from build123d import *

# Parameters (mm, degrees)
BOSS_EXTRUDE1_DEPTH = 0.3
SKETCH2_R           = 0.085
CUT_EXTRUDE1_DEPTH  = 0.3


with BuildPart() as part:
    # Sketch1 → Boss-Extrude1 (new body)
    with BuildSketch(Plane(origin=(0, 0, 0), x_dir=(1, 0, 0), z_dir=(0, 1, 0))):
        with BuildLine():
            Line((0.284268307, -3), (-0.284268307, -3))
            Line((-0.284268307, -3), (-0.123615756, -0.587127878))
            ThreePointArc((-0.123615756, -0.587127878), (-0.6, 0), (-0.123615756, 0.587127878))
            Line((-0.123615756, 0.587127878), (-0.123615756, 14))
            Line((-0.123615756, 14), (0.123615756, 14))
            Line((0.123615756, 14), (0.123615756, 0.587127878))
            ThreePointArc((0.123615756, 0.587127878), (0.6, 0), (0.123615756, -0.587127878))
            Line((0.123615756, -0.587127878), (0.284268307, -3))
        make_face()
    extrude(amount=BOSS_EXTRUDE1_DEPTH)

    # Sketch2 → Cut-Extrude1 (cut)
    with BuildSketch(Plane(origin=(0, 0.3, 0), x_dir=(1, 0, 0), z_dir=(0, 1, 0))):
        Circle(SKETCH2_R)
    extrude(amount=-CUT_EXTRUDE1_DEPTH, mode=Mode.SUBTRACT)


solid = part.part
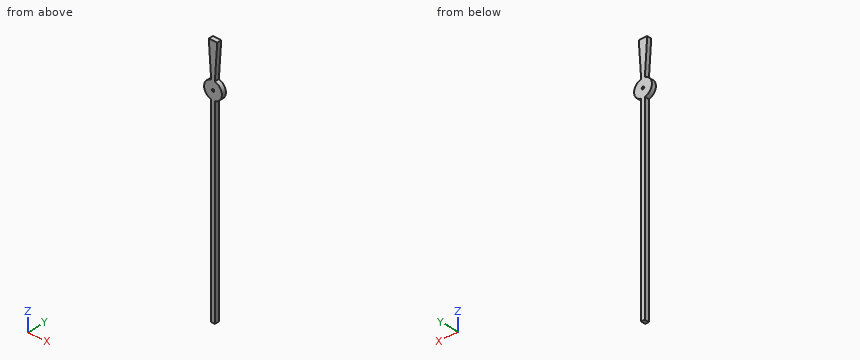
Check sheet for the modelled part. Datum: model origin and axes. Units: mm. Give positions to 0.01 mm unless a question says otherwise; leave off trailing zeros. Order: outer loops, then holes, each group sorted by start corner. A loop starts at its lowest first (then second) coordinate and runs counter-clockwise, first axis right, second up. Notation, with made-up numbers: M 44,79 L 100,79 A16 ccw 100,91 Z; hole C -28.5,-35 d6. An arc over 180 degrees is marked long. Answer as CSV lines item,"result". Start each with the question number.
Item 1: Cross-section at B-B on z = -9. Enter the section's corners in (x, y).
Item 2: Thickness scan on line 1 (Z direction, x = 0, y = 0.25) (3 decimals); line 2 (X direction, y = 0.1, z = 0) (3 decimals); line 3 (X direction, y = 0.1, z = -7.75). Record the ranges inside material, lowest first. Write a range as [from, to].
Item 3: Cross-section at C-C on z = 1. Enter the section's corners in (x, y).
Item 4: Cross-section at A-A on y = 0.2. Enter the section's corners in (x, z) (3 decimals).
Established:
1,outline,"M -0.12,0 L 0.12,0 L 0.12,0.3 L -0.12,0.3 Z"
2,line 1,"z = [-14, -0.085], [0.085, 3]"
2,line 2,"x = [-0.6, -0.085], [0.085, 0.6]"
2,line 3,"x = [-0.12, 0.12]"
3,outline,"M -0.15,0 L 0.15,0 L 0.15,0.3 L -0.15,0.3 Z"
4,outline,"M -0.284,3 L -0.124,0.587 A0.6 ccw -0.124,-0.587 L -0.124,-14 L 0.124,-14 L 0.124,-0.587 A0.6 ccw 0.124,0.587 L 0.284,3 Z; hole C 0,0 d0.17"
